Geometry: final body of the model. Coordinates: model frame, mm. A direction names the side the tool comes from. Round coordinates to 2 decimals unless told otherwise and drop trailing zeros. Loops run counter-clockwise (first coordinate to the right, second up) from the corner with the lowest first, then second, coordinate; pieces in that order, holes last. Notation, with made-up numbers: (-37, 71.5) - (9, 71.5) arc R31 cw to (9, 101.5) - close; hole circle Ø8 at (68, 53). An arc over 180 degrees is marked (long way). Answer as a JSON object with one key per item and string values. Group by question number.
Item 1: Section A-A (x = 0). Return the cut outline in (y, z).
Item 2: Section B-B (y = 0). Return the cut outline in (x, z), plus the area to 3 significant figures.
Item 3: Section D-D (x = -9). Return the cut outline in (y, z), plus the area to 3 significant figures.
Item 4: Section C-C (z = 57.5). Return the cut outline in (x, y), plus the area to 3 significant figures.
Item 5: Line query: line 1 (Z direction, x = -13.5, y = -9); line 2 (Z direction, x = -11, y = -13); line 3 (Y direction, x = -1, z = 60). Output: solid intervals per line, ascending.
Item 6: Reachability of faces 1 (the face through (-0.1, -4.6, 51.1)), 2 (the face through (0, -4.95, 58)), 3 (the face through (-17, 3, 22.1)) from +Z, -Z, +X, -X, +Y, -Y: full face, straight path, thin tool, end or side. Return the list, or none.
Item 7: First-contact query: pin 1 (18.5 mm diameter, centred on x = -2.5, y = 3.5, fed in from -Z); pin 2 (3 mm diameter, centred on x = -6.5, z = 26, fed in from +Y); pin 3 (8 mm diameter, centred on y = 11, z = 21, fed in from -X); pin 4 (12 mm diameter, centred on x = -6.5, y = 14.5, fed in from +Z). Flat tips, straight axial feed; report the tip coordinate or a pass-through.
```python
from build123d import *

# Parameters (mm, degrees)
CROQUIS1_R              = 16.65
SALIENTE_EXTRUIR1_DEPTH = 22.1
CROQUIS2_R              = 18.5
SALIENTE_EXTRUIR3_DEPTH = 22.3
CROQUIS3_R              = 5.95
SALIENTE_EXTRUIR4_DEPTH = 6.7
SALIENTE_EXTRUIR5_DEPTH = 15


with BuildPart() as part:
    # Croquis1 → Saliente-Extruir1 (new body)
    with BuildSketch(Plane.XY):
        Circle(CROQUIS1_R)
    extrude(amount=SALIENTE_EXTRUIR1_DEPTH)

    # Croquis2 → Saliente-Extruir3 (add)
    with BuildSketch(Plane.XY.offset(22.1)):
        Circle(CROQUIS2_R)
    extrude(amount=SALIENTE_EXTRUIR3_DEPTH)

    # Croquis3 → Saliente-Extruir4 (add)
    with BuildSketch(Plane.XY.offset(44.4)):
        with Locations((0, -7.35)):
            Circle(CROQUIS3_R)
    extrude(amount=SALIENTE_EXTRUIR4_DEPTH)

    # Croquis4 → Saliente-Extruir5 (add)
    with BuildSketch(Plane.XY.offset(51.1)):
        with BuildLine():
            Line((-1.8, -4.95), (1.8, -4.95))
            ThreePointArc((1.8, -4.95), (0, -10.35), (-1.8, -4.95))
        make_face()
    extrude(amount=SALIENTE_EXTRUIR5_DEPTH)


solid = part.part
```
Values:
{
 "1": {"outline": "(-18.5, 22.1) - (-16.65, 22.1) - (-16.65, 0) - (16.65, 0) - (16.65, 22.1) - (18.5, 22.1) - (18.5, 44.4) - (-1.4, 44.4) - (-1.4, 51.1) - (-4.95, 51.1) - (-4.95, 66.1) - (-10.35, 66.1) - (-10.35, 51.1) - (-13.3, 51.1) - (-13.3, 44.4) - (-18.5, 44.4) - close"},
 "2": {"outline": "(-18.5, 22.1) - (-16.65, 22.1) - (-16.65, 0) - (16.65, 0) - (16.65, 22.1) - (18.5, 22.1) - (18.5, 44.4) - (-18.5, 44.4) - close", "area": "1,560 mm^2"},
 "3": {"outline": "(-16.16, 22.1) - (-14.01, 22.1) - (-14.01, 0) - (14.01, 0) - (14.01, 22.1) - (16.16, 22.1) - (16.16, 44.4) - (-16.16, 44.4) - close", "area": "1,340 mm^2"},
 "4": {"outline": "(-1.8, -4.95) arc R3 ccw (long way) to (1.8, -4.95) - close", "area": "26.8 mm^2"},
 "5": {"line 1": "z = 0 to 44.4", "line 2": "z = 22.1 to 44.4", "line 3": "y = -10.18 to -4.95"},
 "6": {"face 1": "+Z", "face 2": "+Z, +X, -X, +Y", "face 3": "-Z"},
 "7": {"pin 1": "stops at z = 0", "pin 2": "stops at y = 17.81", "pin 3": "stops at x = -17.06", "pin 4": "stops at z = 44.4"}
}
